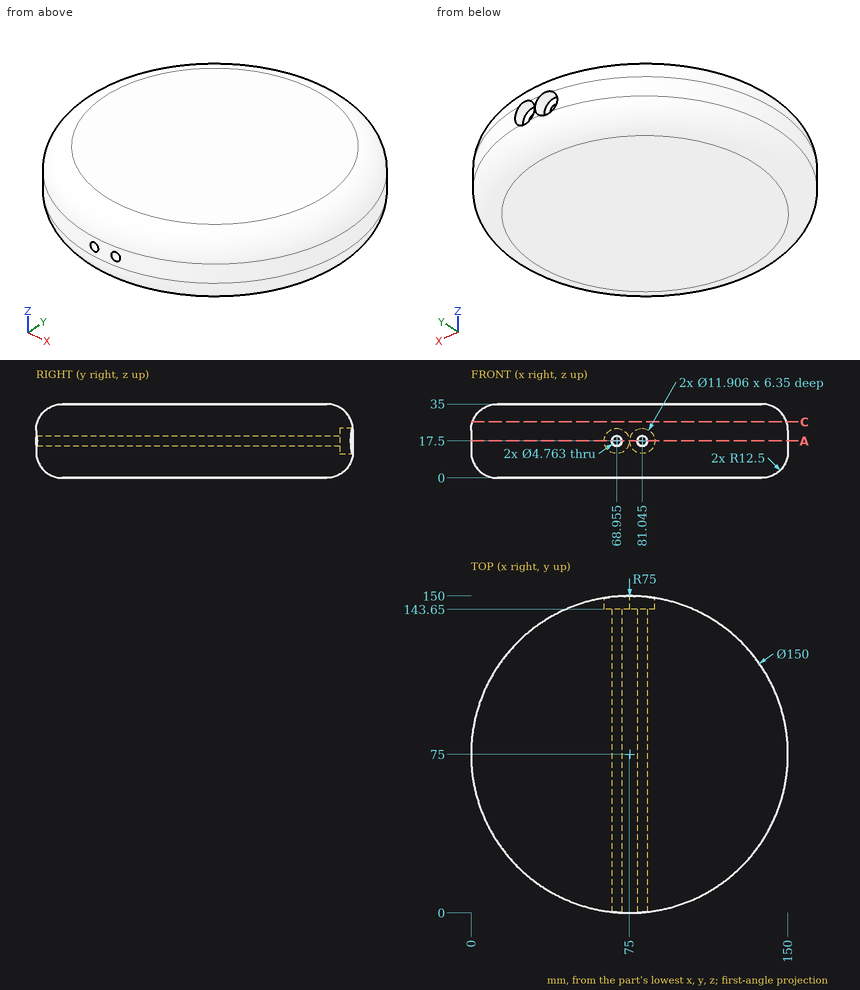
Geometry check sheet. Reference: drawing and pictorial views, mm from the part's lowest x, y, z. Give positions to 0.01 mm unless a question says otherwise; leave off trailing zeros. Loops run counter-clockwise (first coordinate to the right, second up) from the corner with the lowest first, then second, coordinate; pieces in that order, holes last. Notation, with made-up numbers: M 59.5,43.5 L 70.5,43.5 A16 cw 70.5,52.5 Z; hole C -6.75,11 d3. An arc over 180 degrees is marked long. Use a Markdown table: item, result. Add a question column.
Q1. Go/stop test with flat-tipped pins: pin 1 (4.5 mm diameter, centred on x = 81.045, z = 17.5, fed in from -Y); pin 2 (6 mm diameter, centred on y = 112.5, z = 7, fed in from +X); pin 3 (1 mm diameter, centred on y = 94.5, z = 29.5, fed in from +X); pin 4 (7 mm diameter, centred on x = 68.955, z = 17.5, fed in from +Y). Record where each tip stops, or that it passes through.
Q2. Sectioned sample at A-A, the plane z = 17.5. Give the number of separate pieces and of enclosed holes in the cut face, then the cut area to 3 significant figures.
Q3. Scan lines: line 1 along X through (y, z) = (40, 17) (1 decimal); line 2 along X through (y, z) = (113.5, 17.5) (1 decimal); line 3 along Y through (x, z) = (79, 21.5). Record each from-to range of solid material in increasing order. Write a range as [from, to].
Q4. Sectioned sample at C-C, the plane z = 26.5. Record the cut outline in (x, y) (1 decimal).
Verdict:
| question | item | result |
|---|---|---|
| 1 | pin 1 | through |
| 1 | pin 2 | x = 140.65 |
| 1 | pin 3 | x = 145.56 |
| 1 | pin 4 | y = 143.65 |
| 2 | separate pieces | 3 |
| 2 | enclosed holes | 0 |
| 2 | area | 16,200 mm^2 |
| 3 | line 1 | [8.7, 66.6], [71.3, 78.7], [83.4, 141.3] |
| 3 | line 2 | [10.6, 66.6], [71.3, 78.7], [83.4, 139.4] |
| 3 | line 3 | [0.11, 143.65] |
| 4 | outline | C 75,75 d148.7 |
